Input: part model. Units: mm. Frame: model coordinates. A direction names the side the tool comes from. Round coordinates to 2 decimals unless told otherwise and drop trailing zeros. Write each loop counter-clockwise with the first axis right and the second up, starting at its lowest first coordinate (ties: lowest second). Pieces come first, ordered by that corner, then holes. Notation, with made-up numbers: (31, 17.5) - (88, 17.5) arc R15 ccw to (88, 35.5) - close; hole circle Ø5 at (10.5, -21.5). An arc over 180 degrees is marked (long way). One line per item, written item: value. Start each with the question number.
```python
from build123d import *

# Parameters (mm, degrees)
SKETCH_1_R          = 1.65
SKETCH_1_R_2        = 12.15
EXTRUDE_6_DEPTH     = 3
SKETCH_4_W          = 3
SKETCH_4_H          = 30
EXTRUDE_7_DEPTH     = 12
SKETCH_5_R          = 1.65
CUT_EXTRUDE_1_DEPTH = 56
FILLET_6_R          = 2


with BuildPart() as part:
    # 草图1 → 凸台-拉伸6 (new body)
    with BuildSketch(Plane.XY):
        Polygon((0, 30), (0, 0), (56, 0), (56, 30), (47.77634117, 30), (42.77391153, 35.00242964), (13.226088475, 35.00242964), (8.223658835, 30), align=None)
        with Locations((16, 29)):
            Circle(SKETCH_1_R, mode=Mode.SUBTRACT)
        with Locations((40, 29)):
            Circle(SKETCH_1_R, mode=Mode.SUBTRACT)
        with Locations((8.223658835, 6.5)):
            Circle(SKETCH_1_R, mode=Mode.SUBTRACT)
        with Locations((16, 5)):
            Circle(SKETCH_1_R, mode=Mode.SUBTRACT)
        with Locations((8.223658835, 13)):
            Circle(SKETCH_1_R, mode=Mode.SUBTRACT)
        with Locations((40, 5)):
            Circle(SKETCH_1_R, mode=Mode.SUBTRACT)
        with Locations((47.77634117, 6.5)):
            Circle(SKETCH_1_R, mode=Mode.SUBTRACT)
        with Locations((28, 17)):
            Circle(SKETCH_1_R_2, mode=Mode.SUBTRACT)
        with Locations((47.77634117, 13)):
            Circle(SKETCH_1_R, mode=Mode.SUBTRACT)
        with Locations((8.223658835, 19.5)):
            Circle(SKETCH_1_R, mode=Mode.SUBTRACT)
        with Locations((47.77634117, 19.5)):
            Circle(SKETCH_1_R, mode=Mode.SUBTRACT)
    extrude(amount=EXTRUDE_6_DEPTH)

    # 草图4 → 凸台-拉伸7 (add)
    with BuildSketch(Plane.XY.offset(3)):
        with Locations((1.5, 15)):
            Rectangle(SKETCH_4_W, SKETCH_4_H)
        with Locations((54.5, 15)):
            Rectangle(SKETCH_4_W, SKETCH_4_H)
    extrude(amount=EXTRUDE_7_DEPTH)

    # 草图5 → 切除-拉伸1 (cut)
    with BuildSketch(Plane(origin=(56, 0, 0), x_dir=(0, 0, -1), z_dir=(1, 0, 0))):
        with Locations((-11, 18.525)):
            Circle(SKETCH_5_R)
        with BuildLine():
            ThreePointArc((-9.35, 12.4), (-12.166726189, 13.566726189), (-11, 10.75))
            Line((-11, 10.75), (-11, 12.4))
            Line((-11, 12.4), (-9.35, 12.4))
        make_face()
        with BuildLine():
            Line((-11, 12.4), (-11, 10.75))
            ThreePointArc((-11, 10.75), (-9.833273811, 11.233273811), (-9.35, 12.4))
            Line((-9.35, 12.4), (-11, 12.4))
        make_face()
        with BuildLine():
            ThreePointArc((-11, 7.925), (-12.65, 6.275), (-11, 4.625))
            Line((-11, 4.625), (-11, 6.275))
            Line((-11, 6.275), (-11, 7.925))
        make_face()
        with BuildLine():
            Line((-11, 6.275), (-11, 4.625))
            ThreePointArc((-11, 4.625), (-9.833273811, 5.108273811), (-9.35, 6.275))
            ThreePointArc((-9.35, 6.275), (-9.833273811, 7.441726189), (-11, 7.925))
            Line((-11, 7.925), (-11, 6.275))
        make_face()
    extrude(amount=-CUT_EXTRUDE_1_DEPTH, mode=Mode.SUBTRACT)

    # 圆角6
    fillet_6_edges = [part.edges().sort_by_distance(p)[0] for p in [
        (8.223658835, 30, 1.5),
        (13.226088475, 35.00242964, 1.5),
        (42.77391153, 35.00242964, 1.5),
        (47.77634117, 30, 1.5),
        (1.5, 30, 15),
        (1.5, 0, 15),
        (54.5, 30, 15),
        (54.5, 0, 15),
    ]]
    fillet(fillet_6_edges, radius=FILLET_6_R)


solid = part.part
```
Q1. Cut plane C-C, the plane y = 19.5. Output: boundary loops of the cut face in (x, z), and give its area (3 significant figures).
Q2. Cut plane D-D, the plane x = 5. Output: boundary loops of the cut face in (y, z), and give its area (3 significant figures).
Q3. Pull-direction query (Y, two-part tool) for faces 1 (the flat face through (0, 15, 7)), 2 (the flat face through (54, 30, 5)), 3 (the cylindrical face through (48.663, 20.891, 1.479)); classes: pulls with the +Y half, pulls with the -Y half, needs draft (parallel to the pull), parting line crosses it, or undercut.
Q4. Cut plane B-B, the plane z = 7. Output: boundary loops of the cut face in (x, y).
Q5. Material intervals for probe 1 along X at (y, z) = (7.5, 5.25); probe 2 along Z at (x, y) = (42.5, 22), sorted ascending. Write a range as from..to.
Q6. Cut plane A-A, the plane x = 28. Output: boundary loops of the cut face in (y, z), and give its area (3 significant figures).
Q7. Access query for faces 4 (the flat face through (3, 15, 9)), 5 (the cylindrical face through (38.35, 5.07, 1.48)), 6 (the flat face through (2, 30, 5)). Directions: +Z, -Z, +X, -X, +Y, -Y. A direction counts if a zero-diameter tool reaches every point of the face in a straight line with its end or side. Return the directions, or none.
Q8. Contact query for flat-ended pins moving along their axis: pin 1 Ø3.5 at (x, z) = (2.5, 5) entering from +Y; pin 2 Ø5 at (x, z) = (22, 7) entering from -Y; pin 3 Ø3 at (x, y) = (22, 7) entering from +Z. Output: stop coordinate, or through.
A:
1. outline: (0, 0) - (6.57, 0) - (6.57, 3) - (3, 3) - (3, 9.67) - (0, 9.67) - close; (0, 12.33) - (3, 12.33) - (3, 15) - (0, 15) - close; (9.87, 0) - (16.11, 0) - (16.11, 3) - (9.87, 3) - close; (39.89, 0) - (46.13, 0) - (46.13, 3) - (39.89, 3) - close; (49.43, 0) - (56, 0) - (56, 9.67) - (53, 9.67) - (53, 3) - (49.43, 3) - close; (53, 12.33) - (56, 12.33) - (56, 15) - (53, 15) - close
1. area: 133 mm²
2. outline: (0, 0) - (30, 0) - (30, 3) - (0, 3) - close
2. area: 90.0 mm²
3. face 1: needs draft
3. face 2: pulls with the +Y half
3. face 3: undercut
4. outline: (0, 0) - (3, 0) - (3, 30) - (0, 30) - close; (53, 0) - (56, 0) - (56, 30) - (53, 30) - close
5. probe 1: x = 0..3, 53..56
5. probe 2: z = 0..3
6. outline: (0, 0) - (4.85, 0) - (4.85, 3) - (0, 3) - close; (29.15, 0) - (35, 0) - (35, 3) - (29.15, 3) - close
6. area: 32.1 mm²
7. face 4: +Z, +Y, -Y
7. face 5: +Z, -Z
7. face 6: +Z, -Z, -X, +Y
8. pin 1: stops at y = 30
8. pin 2: passes through
8. pin 3: stops at z = 3
